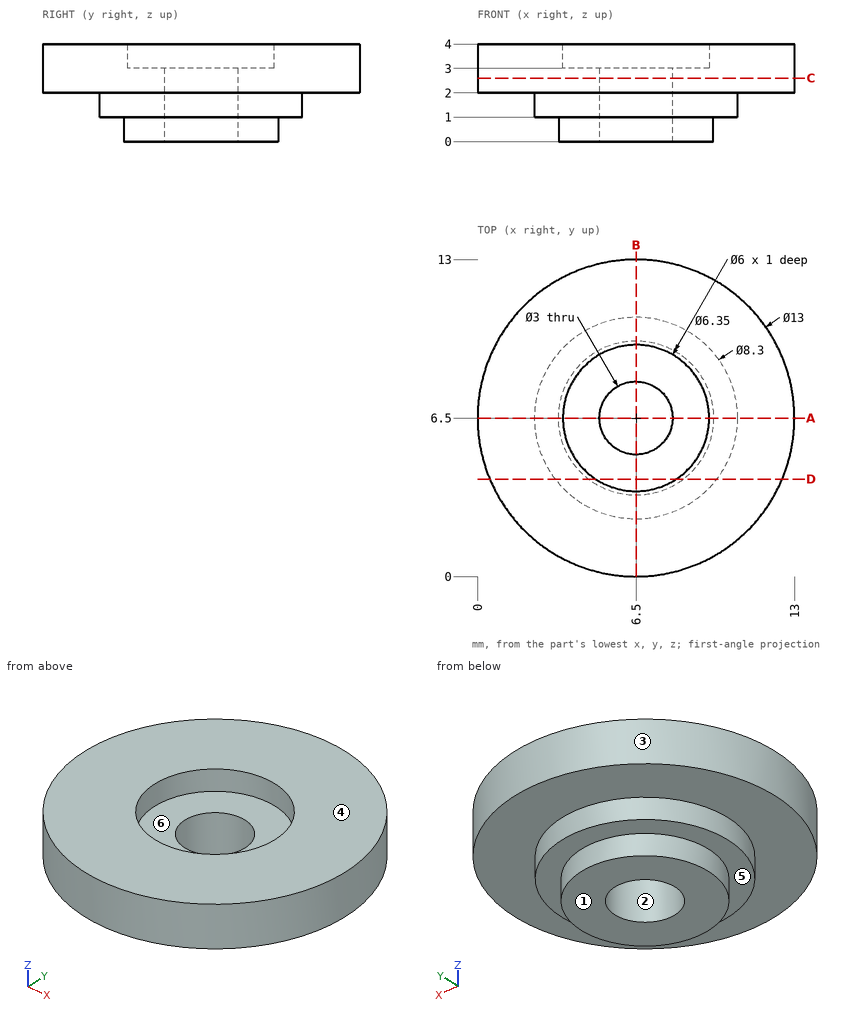
Job drawing, mm, ordinate dimensions from the low corner. One solid piece. A direction names the side the tool comes from. Coordinates: 2 decimals unless noted, no trailing zeros. Write each loop counter-clockwise with the first axis right and the second up, starting at its lowest first coordinate (ties: lowest second). Pieces come first, ordered by that corner, then holes. Notation, with made-up numbers: M 81,3 L 101,3 A19 cw 101,39 Z; hole C 54.5,-33.75 d9. An arc over 180 degrees is marked long. Answer as a JSON object with one key per item and string values. Group by question number.
1) Tool access for the marked faces 4, 5 and 6: list every direction of +Z, -Z, +X, -X, +Y, -Y with a clear straight run to the whole face (end or side of a thin tool).
2) Pin check, flat tips, straight feed: pin 1 Ø1 at (y, z) = (9.5, 3) entering from -X; pin 2 Ø5 at (x, y) = (6.5, 6.5) entering from -Z; pin 3 Ø5 at (x, y) = (6.5, 6.5) entering from +Z; pin 4 Ø1.5 at (x, z) = (7.5, 1) entering from -Y. Stop position of each tip, or through.
3) Wall check: line 1 (X direction, y = 6.5, z = 1.4); line 2 (Y direction, x = 6.5, z = 3.5); line 3 (Y direction, x = 6.5, z = 0.85) (3 decimals). Give the ranges that are in metal, low to high. Write a range as from..to.
4) Saw through at A-A (y = 6.5). Write the cut outline in (x, z) (3 decimals), plus the area to 4 significant figures.
5) Mould opens along X. For the marked faces 1, 2 and 3 say: +X half, -X half, draft (parallel to the pull), parting line (faces both ways), or undercut.
6) Saw through at D-D (y = 4). Write the cut outline in (x, z), plus the area to 3 significant figures.
7) Saw through at C-C (z = 2.6). Write the cut outline in (x, y), plus the area to 3 significant figures.
Values follow:
{
 "1": {"face 4": "+Z, +X, -X, +Y, -Y", "face 5": "-Z", "face 6": "+Z"},
 "2": {"pin 1": "stops at x = 0.5", "pin 2": "stops at z = 0", "pin 3": "stops at z = 3", "pin 4": "stops at y = 2.36"},
 "3": {"line 1": "x = 2.35..5, 8..10.65", "line 2": "y = 0..3.5, 9.5..13", "line 3": "y = 3.325..5, 8..9.675"},
 "4": {"outline": "M 0,2 L 2.35,2 L 2.35,1 L 3.325,1 L 3.325,0 L 5,0 L 5,3 L 3.5,3 L 3.5,4 L 0,4 Z; M 8,0 L 9.675,0 L 9.675,1 L 10.65,1 L 10.65,2 L 13,2 L 13,4 L 9.5,4 L 9.5,3 L 8,3 Z", "area": "25.65 mm2"},
 "5": {"face 1": "draft", "face 2": "undercut", "face 3": "parting line"},
 "6": {"outline": "M 0.5,2 L 3.19,2 L 3.19,1 L 4.54,1 L 4.54,0 L 8.46,0 L 8.46,1 L 9.81,1 L 9.81,2 L 12.5,2 L 12.5,4 L 8.16,4 L 8.16,3 L 4.84,3 L 4.84,4 L 0.5,4 Z", "area": "31.2 mm2"},
 "7": {"outline": "C 6.5,6.5 d13; hole C 6.5,6.5 d3", "area": "126 mm2"}
}
